from build123d import *

# Parameters (mm, degrees)
SKETCH1_W                    = 44.45
SKETCH1_H                    = 12.7
BOSS_EXTRUDE4_DEPTH          = 6.35
FILLET3_R                    = 6.35
F_18_0_1695_DIAMETER_HOLE2_D = 4.3053
CUT_EXTRUDE1_DEPTH           = 6.35


with BuildPart() as part:
    # Sketch1 → Boss-Extrude4 (new body)
    with BuildSketch(Plane(origin=(0, 0, 0), x_dir=(1, 0, 0), z_dir=(0, 1, 0))):
        Rectangle(SKETCH1_W, SKETCH1_H)
    extrude(amount=BOSS_EXTRUDE4_DEPTH)

    # Fillet3
    fillet3_edges = [part.edges().sort_by_distance(p)[0] for p in [
        (22.225, 3.175, -6.35),
        (22.225, 3.175, 6.35),
        (-22.225, 3.175, -6.35),
        (-22.225, 3.175, 6.35),
    ]]
    fillet(fillet3_edges, radius=FILLET3_R - 0.0001)  # a hair under: the kernel refuses the full size

    # #18 (0.1695) Diameter Hole2 (through all)
    with Locations(Plane(origin=(0, 6.35, 0), x_dir=(1, 0, 0), z_dir=(0, 1, 0))):
        with Locations((-15.875, 0), (15.875, 0)):
            Hole(F_18_0_1695_DIAMETER_HOLE2_D / 2)

    # Sketch10 → Cut-Extrude1 (cut)
    with BuildSketch(Plane(origin=(0, 6.35, 0), x_dir=(1, 0, 0), z_dir=(0, 1, 0))):
        with BuildLine():
            Line((-8.255, 3.96875), (8.255, 3.96875))
            ThreePointArc((8.255, 3.96875), (9.153025612, 3.596775612), (9.525, 2.69875))
            Line((9.525, 2.69875), (9.525, -2.69875))
            ThreePointArc((9.525, -2.69875), (9.153025612, -3.596775612), (8.255, -3.96875))
            Line((8.255, -3.96875), (-8.255, -3.96875))
            ThreePointArc((-8.255, -3.96875), (-9.153025612, -3.596775612), (-9.525, -2.69875))
            Line((-9.525, -2.69875), (-9.525, 2.69875))
            ThreePointArc((-9.525, 2.69875), (-9.153025612, 3.596775612), (-8.255, 3.96875))
        make_face()
    extrude(amount=-CUT_EXTRUDE1_DEPTH, mode=Mode.SUBTRACT)


solid = part.part
For this review, take the finished solid that the model builds, in its own axes (mm). A direction names the side the tool comes from. Round coordinates to 2 decimals unless told otherwise and drop trailing zeros. Order: outer loops, then holes, each group sorted by start corner. A loop starts at its lowest first (then second) coordinate and runs counter-clockwise, first axis right, second up. Notation, with made-up numbers: (37, 63.5) -> (54, 63.5) arc R37 cw to (54, 101.5) -> close; hole circle Ø6 at (4.25, -30.5). An arc over 180 degrees is marked (long way). Write item = value, one per line. Start each with the question number.
1) Take a section at B-B on z = -0.75. State the section outline as (x, y) points (3 decimals), plus the area to 3 significant figures.
2) The part is to be moulded in two halves that separate along X. For faces 1 (the face through (-20.414, 3.219, 4.441)), 2 (the face through (-9.525, 3, 0)), 3 (the face through (-0.3, 0, -4.3)), say which applies: +X half, -X half, draft (parallel to the pull), parting line (faces both ways), or undercut.
3) Tool access review of faces 4 (the face through (20.414, 3.219, -4.441)), 5 (the face through (-9.14, 3.22, 3.61)): name each direction out of +Z, -Z, +X, -X, +Y, -Y from which nothing blocks a thin tool from reaching the whole face with its end or side.
4) Take a section at C-C on x = 17. State the section outline as (y, z) points.
5) To check wall thickness, follow line 1 (Z direction, x = -2.5, y = 5); line 2 (X direction, y = 0.5, z = -0.75) (3 decimals); line 3 (Z direction, x = -9, y = 5). State the ranges of each line that lie inside material, in increasing order. Write a range as from..to.
6) Take a section at D-D on x = -14.5. State the section outline as (y, z) points.
7) Take a section at A-A on y = 3. Count the separate pieces of the cut face and the enclosed holes in it, plus the area to 3 significant figures.
8) Insertion check: pin 1 (1 mm diameter, centred on y = 4.5, z = 3.5, fed in from -X); pin 2 (3 mm diameter, centred on y = 5.5, z = -4.5, fed in from +X). Each pin has a flat end and moves straight along its axis. Give the tip position at first contact, or say it passes through.
Verdict:
q1.outline = (-22.181, 0) -> (-17.893, 0) -> (-17.893, 6.35) -> (-22.181, 6.35) -> close; (-13.857, 0) -> (-9.525, 0) -> (-9.525, 6.35) -> (-13.857, 6.35) -> close; (9.525, 0) -> (13.857, 0) -> (13.857, 6.35) -> (9.525, 6.35) -> close; (17.893, 0) -> (22.181, 0) -> (22.181, 6.35) -> (17.893, 6.35) -> close
q1.area = 109 mm2
q2.face_1 = -X half
q2.face_2 = undercut
q2.face_3 = draft
q3.face_4 = -Z, +X, +Y, -Y
q3.face_5 = +Y, -Y
q4.outline = (0, -6.25) -> (6.35, -6.25) -> (6.35, -1.84) -> (0, -1.84) -> close; (0, 1.84) -> (6.35, 1.84) -> (6.35, 6.25) -> (0, 6.25) -> close
q5.line_1 = -6.35..-3.97, 3.97..6.35
q5.line_2 = -22.181..-17.893, -13.857..-9.525, 9.525..13.857, 17.893..22.181
q5.line_3 = -6.35..-3.73, 3.73..6.35
q6.outline = (0, -6.35) -> (6.35, -6.35) -> (6.35, -1.66) -> (0, -1.66) -> close; (0, 1.66) -> (6.35, 1.66) -> (6.35, 6.35) -> (0, 6.35) -> close
q7.separate_pieces = 1
q7.enclosed_holes = 3
q7.area = 351 mm2
q8.pin_1 = -21.47
q8.pin_2 = 21.47
